Read the model definition and answer for the solid it produces. Units are mm, in the model's axes. A direction names the side the tool comes from. Coordinates: 2 decimals unless noted, no trailing zeros. Order: outer loops, then holes, each group sorted by start corner. A loop starts at its lowest first (then second) coordinate and runs counter-clockwise, first axis right, second up. Notation, with made-up numbers: M -38,58 L -11,58 A23 ccw -11,81 Z; hole C 23.25,67.25 d4. An arc over 180 degrees is marked long. Put each result on its own line as item: value.
from build123d import *

# Parameters (mm, degrees)
CROQUIS1_W                        = 21.8
CROQUIS1_H                        = 30
SALIENTE_EXTRUIR1_DEPTH           = 21.8
CROQUIS6_R                        = 2
CORTAR_EXTRUIR2_DEPTH             = 21.8
CORTAR_EXTRUIR4_REACH             = 45.017
CROQUIS11_R                       = 3.5
CROQUIS11_W                       = 3.4
CROQUIS11_H                       = 8.4
CORTAR_EXTRUIR4_DIRECTION_2_DEPTH = 3.5
REDONDEO1_R                       = 5
CROQUIS13_R                       = 3.5
CORTAR_EXTRUIR6_DEPTH             = 3.5
CROQUIS16_W                       = 10.1
CROQUIS16_H                       = 20.1
CORTAR_EXTRUIR7_DEPTH             = 2
CROQUIS17_W                       = 10.1
CROQUIS17_H                       = 20.1
CORTAR_EXTRUIR8_DEPTH             = 2
CORTAR_EXTRUIR9_START             = -3.5
CROQUIS7_R                        = 3.5
CORTAR_EXTRUIR9_DEPTH             = 3.5


with BuildPart() as part:
    # Croquis1 → Saliente-Extruir1 (new body)
    with BuildSketch(Plane(origin=(0, 0, 0), x_dir=(0, 0, -1), z_dir=(1, 0, 0))):
        with Locations((-10.9, -15)):
            Rectangle(CROQUIS1_W, CROQUIS1_H)
    extrude(amount=SALIENTE_EXTRUIR1_DEPTH)

    # Croquis6 → Cortar-Extruir2 (cut)
    with BuildSketch(Plane.ZY):
        with Locations((10.9, -22)):
            Circle(CROQUIS6_R)
        with Locations((10.9, -7)):
            Circle(CROQUIS6_R)
    extrude(amount=-CORTAR_EXTRUIR2_DEPTH, mode=Mode.SUBTRACT)

    # Cortar-Extruir4: up to this face of the body (flat: up to its plane)
    cortar_extruir4_end = Plane(part.part.faces().sort_by_distance((10.9, 0, 10.9))[0])
    # Croquis11 → Cortar-Extruir4 (cut, up to the picked face)
    with BuildSketch(Plane.XZ.offset(30), mode=Mode.PRIVATE) as cortar_extruir4_sk1:
        with Locations(Location((13.4, 10.9, 0), (0, 0, 270))):
            Circle(CROQUIS11_R)
    cortar_extruir4_tool1 = split(extrude(cortar_extruir4_sk1.sketch, amount=-CORTAR_EXTRUIR4_REACH, mode=Mode.PRIVATE), bisect_by=cortar_extruir4_end, keep=Keep.BOTH, mode=Mode.PRIVATE)
    # Croquis11 → Cortar-Extruir4 (cut, up to the picked face)
    with BuildSketch(Plane.XZ.offset(30), mode=Mode.PRIVATE) as cortar_extruir4_sk2:
        with Locations((7.2, 10.9)):
            Rectangle(CROQUIS11_W, CROQUIS11_H)
    cortar_extruir4_tool2 = split(extrude(cortar_extruir4_sk2.sketch, amount=-CORTAR_EXTRUIR4_REACH, mode=Mode.PRIVATE), bisect_by=cortar_extruir4_end, keep=Keep.BOTH, mode=Mode.PRIVATE)
    add(cortar_extruir4_tool1.solids().sort_by(Axis((13.4, -30, 10.9), (0, 1, 0)))[0], mode=Mode.SUBTRACT)
    add(cortar_extruir4_tool2.solids().sort_by(Axis((7.2, -30, 10.9), (0, 1, 0)))[0], mode=Mode.SUBTRACT)

    # Croquis11 → Cortar-Extruir4 direction 2 (cut)
    with BuildSketch(Plane.XZ.offset(30)):
        with Locations(Location((13.4, 10.9, 0), (0, 0, 270))):
            Circle(CROQUIS11_R)
        with Locations((7.2, 10.9)):
            Rectangle(CROQUIS11_W, CROQUIS11_H)
    extrude(amount=CORTAR_EXTRUIR4_DIRECTION_2_DEPTH, mode=Mode.SUBTRACT)

    # Redondeo1
    # the kernel refuses this fillet: 5 mm, written as the material it takes off along each edge
    with BuildSketch(Plane(origin=(21.8, -30, 34.3), x_dir=(0, 1, 0), z_dir=(0, 0, -1)), Plane(origin=(0, 0, -12.5), x_dir=(1, 0, 0), z_dir=(0, 0, 1))) as redondeo1_piece_1:
        with BuildLine():
            CenterArc((REDONDEO1_R, -REDONDEO1_R), REDONDEO1_R, 90, 90)
            Line((0, -REDONDEO1_R), (0, 0))
            Line((0, 0), (REDONDEO1_R, 0))
        make_face()
    extrude(amount=46.8, mode=Mode.SUBTRACT)
    with BuildSketch(Plane(origin=(21.8, 0, -12.5), x_dir=(-1, 0, 0), z_dir=(0, 0, 1)), Plane(origin=(0, -30, 34.3), x_dir=(0, 1, 0), z_dir=(0, 0, -1))) as redondeo1_piece_2:
        with BuildLine():
            CenterArc((REDONDEO1_R, REDONDEO1_R), REDONDEO1_R, 180, 90)
            Line((0, REDONDEO1_R), (0, 0))
            Line((0, 0), (REDONDEO1_R, 0))
        make_face()
    extrude(amount=46.8, mode=Mode.SUBTRACT)

    # Croquis13 → Cortar-Extruir6 (cut)
    with BuildSketch(Plane.ZY):
        with Locations((10.9, -7)):
            Circle(CROQUIS13_R)
        with Locations(Location((10.9, -22, 0), (0, 0, 301.002719134))):
            Circle(CROQUIS13_R)
    extrude(amount=-CORTAR_EXTRUIR6_DEPTH, mode=Mode.SUBTRACT)

    # Croquis16 → Cortar-Extruir7 (cut)
    with BuildSketch(Plane.XY.offset(21.8)):
        with Locations((10.9, -15)):
            Rectangle(CROQUIS16_W, CROQUIS16_H)
    extrude(amount=-CORTAR_EXTRUIR7_DEPTH, mode=Mode.SUBTRACT)

    # Croquis17 → Cortar-Extruir8 (cut)
    with BuildSketch(Plane(origin=(0, 0, 0), x_dir=(-1, 0, 0), z_dir=(0, 0, -1))):
        with Locations((-10.9, -15)):
            Rectangle(CROQUIS17_W, CROQUIS17_H)
    extrude(amount=-CORTAR_EXTRUIR8_DEPTH, mode=Mode.SUBTRACT)

    # Croquis7 → Cortar-Extruir9 (cut)
    with BuildSketch(Plane(origin=(21.8, 0, 0), x_dir=(0, 0, -1), z_dir=(1, 0, 0)).offset(CORTAR_EXTRUIR9_START)):
        with Locations(Location((-10.9, -22, 0), (0, 0, 238.997280866))):
            Circle(CROQUIS7_R)
        with Locations(Location((-10.9, -7, 0), (0, 0, 180))):
            Circle(CROQUIS7_R)
    extrude(amount=CORTAR_EXTRUIR9_DEPTH, mode=Mode.SUBTRACT)


solid = part.part
Q1. For a pull along Y with two mould halves and no side action, classify faces 6 (the face through (9.5, -30, 11.1)), 7 (the face through (1.73, -25.46, 11.42)), 8 (the face through (12.059, -15.21, 7.667)) as +Y half, -Y half, draft (parallel to the pull), parting line (faces both ways), or undercut.
Answers below:
face 6: -Y half
face 7: undercut
face 8: draft
Q2. Given pin 1 (4.5 mm diameter, centred on y = -7, z = 10.9, fed in from -X); pin 2 (10 mm diameter, centred on x = 13, z = 19.5, fed in from +Y); pin 3 (2.5 mm diameter, centred on x = 7.5, y = -15.5, fed in from -Z); pin 4 (6.5 mm diameter, centred on y = -22, z = 10.9, fed in from +X), each flat-ended and moving along its own axis, determine where each tip first touches the part or whether it passes through.
Answers below:
pin 1: stops at x = 3.5
pin 2: stops at y = 0
pin 3: stops at z = 2
pin 4: stops at x = 18.3
Q3. Find section A-A on x = 13.4. Write down the section's boundary in (y, z), plus the area to 3 significant figures.
Answers below:
outline: M -30,0 L -25.05,0 L -25.05,2 L -4.95,2 L -4.95,0 L 0,0 L 0,7.4 L -30,7.4 Z; M -30,14.4 L 0,14.4 L 0,21.8 L -4.95,21.8 L -4.95,19.8 L -25.05,19.8 L -25.05,21.8 L -30,21.8 Z
area: 364 mm^2
Q4. Find section D-D on x = 19.75. Write down the section's boundary in (y, z).
Answers below:
outline: M -29.04,0 L -0.96,0 L -0.96,21.8 L -29.04,21.8 Z; hole C -22,10.9 d7; hole C -7,10.9 d7
Q5. Consider line 1 along Y through (x, z) = (17, 10.9); line 2 along X through (y, z) = (-5, 14.75); line 3 along Z through (x, y) = (6.5, -11.5). Determine where each line is inside the solid, lowest interval first.
Answers below:
line 1: y = -30 to -24, -20 to -9, -5 to 0
line 2: x = 0 to 5.5, 8.9 to 21.8
line 3: z = 2 to 6.7, 15.1 to 19.8
Q6. Find section B-B on y = -18. Write down the section's boundary in (x, z).
Answers below:
outline: M 0,0 L 5.85,0 L 5.85,2 L 15.95,2 L 15.95,0 L 21.8,0 L 21.8,21.8 L 15.95,21.8 L 15.95,19.8 L 5.85,19.8 L 5.85,21.8 L 0,21.8 Z; hole M 5.5,6.7 L 8.9,6.7 L 8.9,15.1 L 5.5,15.1 Z; hole C 13.4,10.9 d7
Q7. Find section C-C on z = 5.5. Write down the section's boundary in (x, y).
Answers below:
outline: M 0,-25 A5 ccw 5,-30 L 16.8,-30 A5 ccw 21.8,-25 L 21.8,-5 A5 ccw 16.8,0 L 5,0 A5 ccw 0,-5 Z
Q8. A tool of negligible diameter and unlimited length cuts with its end or side. For faces 1 (the face through (11, -15, 19.8)), 2 (the face through (5.5, -15, 11)), 3 (the face through (1.726, -10.417, 10.141)), 4 (the face through (18.3, -23, 13)), 5 (the face through (11, -15, 2)), from which of +Z, -Z, +X, -X, +Y, -Y can it reach the whole face along a straight path? Write none if from no direction.
Answers below:
face 1: +Z
face 2: +Y, -Y
face 3: -X
face 4: +X
face 5: -Z
